from build123d import *

# Parameters (mm, degrees)
SKETCH1_R               = 3.2
BOSS_EXTRUDE1_DEPTH     = 3
SKETCH1_3_R             = 3.2
SKETCH1_3_R_2           = 1.6
BOSS_EXTRUDE2_DEPTH     = 3
BOSS_EXTRUDE3_OUTLINE_W = 23.618802154
BOSS_EXTRUDE3_OUTLINE_H = 3
BOSS_EXTRUDE3_DEPTH     = 10.6
SKETCH3_R               = 1.2
CUT_EXTRUDE4_DEPTH      = 3
SKETCH1_7_W             = 1.759401077
SKETCH1_7_H             = 1.440598923
BOSS_EXTRUDE5_DEPTH     = 5
CHAMFER1_SIZE           = 1.44
CHAMFER2_SIZE           = 3
BOSS_EXTRUDE6_DEPTH     = 2.8
FILLET1_R               = 2


# Read off the part's stored shape, not the designer's step: Boss-Extrude3
with BuildPart() as part:
    # Sketch1 → Boss-Extrude1 (new body)
    with BuildSketch(Plane(origin=(0, 0, 0), x_dir=(1, 0, 0), z_dir=(0, 1, 0))):
        Polygon((11.809401077, 3.2), (10.05, 3.2), (10.05, 6.2), (-10.05, 6.2), (-10.05, 3.2), (-11.809401077, 3.2), (-11.809401077, 1.759401077), (-10.05, 0), (-10.05, -4.6), (10.05, -4.6), (10.05, 0), (11.809401077, 1.759401077), align=None)
        with Locations(Location((-4.05, 0, 0), (0, 0, 270))):
            Circle(SKETCH1_R, mode=Mode.SUBTRACT)
        with Locations(Location((4.05, 0, 0), (0, 0, 270))):
            Circle(SKETCH1_R, mode=Mode.SUBTRACT)
    extrude(amount=BOSS_EXTRUDE1_DEPTH)

    # Sketch1<3> → Boss-Extrude2 (add)
    # profile 1 of 2: a face of its own
    with BuildSketch(Plane(origin=(0, 0, 0), x_dir=(1, 0, 0), z_dir=(0, 1, 0))):
        with Locations((-4.05, 0)):
            Circle(SKETCH1_3_R)
        with Locations(Location((-4.05, 0, 0), (0, 0, 270))):
            Circle(SKETCH1_3_R_2, mode=Mode.SUBTRACT)
    # profile 2 of 2: a face of its own
    with BuildSketch(Plane(origin=(0, 0, 0), x_dir=(1, 0, 0), z_dir=(0, 1, 0))):
        with Locations((4.05, 0)):
            Circle(SKETCH1_3_R)
        with Locations(Location((4.05, 0, 0), (0, 0, 270))):
            Circle(SKETCH1_3_R_2, mode=Mode.SUBTRACT)
    extrude(amount=BOSS_EXTRUDE2_DEPTH)

    # Boss-Extrude3 outline → Boss-Extrude3 (add)
    with BuildSketch(Plane(origin=(0, 0, 0), x_dir=(1, 0, 0), z_dir=(0, 1, 0))):
        with Locations((0, 4.7)):
            Rectangle(BOSS_EXTRUDE3_OUTLINE_W, BOSS_EXTRUDE3_OUTLINE_H)
    extrude(amount=BOSS_EXTRUDE3_DEPTH)

    # Sketch3 → Cut-Extrude4 (cut)
    with BuildSketch(Plane(origin=(0, 0, -6.2), x_dir=(-1, 0, 0), z_dir=(0, 0, -1))):
        with Locations((-7.5, 7)):
            Circle(SKETCH3_R)
        with Locations((7.5, 7)):
            Circle(SKETCH3_R)
        with BuildLine():
            Line((-6.651471863, 7.848528137), (-7.5, 8.697056275))
            Line((-7.5, 8.697056275), (-8.348528137, 7.848528137))
            ThreePointArc((-8.348528137, 7.848528137), (-7.5, 8.2), (-6.651471863, 7.848528137))
        make_face()
        with BuildLine():
            Line((8.348528137, 7.848528137), (7.5, 8.697056275))
            Line((7.5, 8.697056275), (6.651471863, 7.848528137))
            ThreePointArc((6.651471863, 7.848528137), (7.5, 8.2), (8.348528137, 7.848528137))
        make_face()
    extrude(amount=-CUT_EXTRUDE4_DEPTH, mode=Mode.SUBTRACT)

    # Sketch1<7> → Boss-Extrude5 (add)
    with BuildSketch(Plane(origin=(0, 0, 0), x_dir=(1, 0, 0), z_dir=(0, 1, 0))):
        with Locations((-10.929700539, 2.479700539)):
            Rectangle(SKETCH1_7_W, SKETCH1_7_H)
        with Locations((10.929700539, 2.479700539)):
            Rectangle(SKETCH1_7_W, SKETCH1_7_H)
    extrude(amount=BOSS_EXTRUDE5_DEPTH)

    # Chamfer1
    chamfer1_edges = [part.edges().sort_by_distance(p)[0] for p in [
        (-10.929700538, 5, -1.759401077),
        (10.929700538, 5, -1.759401077),
    ]]
    chamfer(chamfer1_edges, length=CHAMFER1_SIZE)

    # Chamfer2
    chamfer2_edges = [part.edges().sort_by_distance(p)[0] for p in [
        (-11.809401077, 10.6, -4.7),
        (11.809401077, 10.6, -4.7),
    ]]
    chamfer(chamfer2_edges, length=CHAMFER2_SIZE)

    # Sketch1<8> → Boss-Extrude6 (add)
    with BuildSketch(Plane(origin=(0, 0, 0), x_dir=(1, 0, 0), z_dir=(0, 1, 0))):
        Polygon((-11.809401077, 9.2), (-11.809401077, 6.2), (-10.05, 6.2), (10.05, 6.2), (11.809401077, 6.2), (11.809401077, 9.2), align=None)
    extrude(amount=BOSS_EXTRUDE6_DEPTH)

    # Fillet1
    fillet1_edges = [part.edges().sort_by_distance(p)[0] for p in [
        (11.809401077, 1.4, -9.2),
        (-11.809401077, 1.4, -9.2),
    ]]
    fillet(fillet1_edges, radius=FILLET1_R)


solid = part.part
CAD build for the part. Positions are in the model's coordinates, mm. A direction names the side the tool comes from. Give positions to 0.01 mm unless a question says otherwise; leave off trailing zeros. Loops run counter-clockwise (first coordinate to the right, second up) from the corner with the lowest first, then second, coordinate; pieces in that order, holes last. Notation, with made-up numbers: M -21.75,27.5 L 25.25,27.5 A25 ccw 25.25,59.5 Z; hole C 7.25,38 d1. An arc over 180 degrees is marked long. Answer in a Markdown table with one row per item. Add a question column.
Item 1: Drop flat-ended pins along their axis: P1, Ø5, axis at x = -4.05, z = 0, coming from the +Y side; P2, Ø1.5, axis at x = -3.5, z = -7, coming from the +Y side; P3, Ø3, axis at x = 7.5, y = 7, coming from the +Z side. Give the stop position or say it passes through.
Item 2: Tool access for faces 4 (the face through (10.33, 9.08, -4.68)), 5 (the face through (10.05, 4, -3)), 6 (the face through (0, 2.8, -8)), 7 (the face through (-7.082, 8.279, -4.721)): list every direction of +Z, -Z, +X, -X, +Y, -Y with a clear straight run to the whole face (end or side of a thin tool).
Item 3: Band-saw the part on C-C on x = 4.75. Give the cut face in (y, z).
Item 4: Band-saw the part on B-B on y = 7. Give the cut face in (x, z), then the cut area to 3 significant figures.
Item 5: Band-saw the part on A-A on y = 2.5. Give the cut face in (x, z), then the cut area to 3 significant figures.
Item 6: Band-saw the part on D-D on z = -4.5. Give the cut face in (x, y).
Item 7: Mould opens along Z. For faces 1 (the face through (0, 3, 1)), 2 (the face through (-10.94, 1.48, -0.89)), 3 (the face through (2.49, 1.48, -0.35)) say: +Z half, -Z half, draft (parallel to the pull), parting line (faces both ways), or undercut.
Item 8: Probe probe 1 along X at (y, z) = (7, -4.15); probe 2 along X at (y, z) = (0.5, -0.5); probe 3 along Y at (x, z) = (8.5, -0.5). List the from-to ranges inside material, lowest first.
Reply:
| question | item | result |
|---|---|---|
| 1 | P1 | stops at y = 3 |
| 1 | P2 | stops at y = 2.8 |
| 1 | P3 | stops at z = -3.2 |
| 2 | face 4 | +Z, -Z, +X, +Y |
| 2 | face 5 | +Z, +Y |
| 2 | face 6 | -Z, +X, -X, +Y |
| 2 | face 7 | +Z, -Z |
| 3 | outline | M 0,-9.2 L 2.8,-9.2 L 2.8,-6.2 L 10.6,-6.2 L 10.6,-3.2 L 3,-3.2 L 3,-1.44 L 0,-1.44 Z; M 0,1.44 L 3,1.44 L 3,4.6 L 0,4.6 Z |
| 4 | outline | M -11.81,-6.2 L -8.7,-6.2 L -8.7,-3.2 L -11.81,-3.2 Z; M -6.3,-6.2 L 6.3,-6.2 L 6.3,-3.2 L -6.3,-3.2 Z; M 8.7,-6.2 L 11.81,-6.2 L 11.81,-3.2 L 8.7,-3.2 Z |
| 4 | area | 56.5 mm^2 |
| 5 | outline | M -11.81,-7.2 A2 ccw -9.81,-9.2 L 9.81,-9.2 A2 ccw 11.81,-7.2 L 11.81,-1.76 L 10.05,0 L 10.05,4.6 L -10.05,4.6 L -10.05,0 L -11.81,-1.76 Z; hole C -4.05,0 d3.2; hole C 4.05,0 d3.2 |
| 5 | area | 289 mm^2 |
| 6 | outline | M -11.81,0 L 11.81,0 L 11.81,7.6 L 8.81,10.6 L -8.81,10.6 L -11.81,7.6 Z; hole M -8.35,7.85 A1.2 ccw long -6.65,7.85 L -7.5,8.7 Z; hole M 6.65,7.85 A1.2 ccw long 8.35,7.85 L 7.5,8.7 Z |
| 7 | face 1 | draft |
| 7 | face 2 | +Z half |
| 7 | face 3 | undercut |
| 8 | probe 1 | x = -11.81 to -8.7, -6.3 to 6.3, 8.7 to 11.81 |
| 8 | probe 2 | x = -10.55 to -5.57, -2.53 to 2.53, 5.57 to 10.55 |
| 8 | probe 3 | y = 0 to 3 |
